Source: three-view drawing plus pictorial views. Frame: mm from the lowest corner of the part. A direction names the side the tool comes from. Give positions to 0.01 mm unless a question says otherwise; leave off trailing zeros. Order: outer loops, then holes, each group sorted by start corner. A loop starts at its lowest first (then second) coordinate and runs counter-clockwise, first axis right, second up. Notation, with made-up numbers: M 25,-22.5 L 67,-22.5 A5 ccw 67,-16.5 Z; hole C 59.25,24 d2. An arc over 180 degrees is marked long. Use CSV: the item, a comma, the result in double quotes.
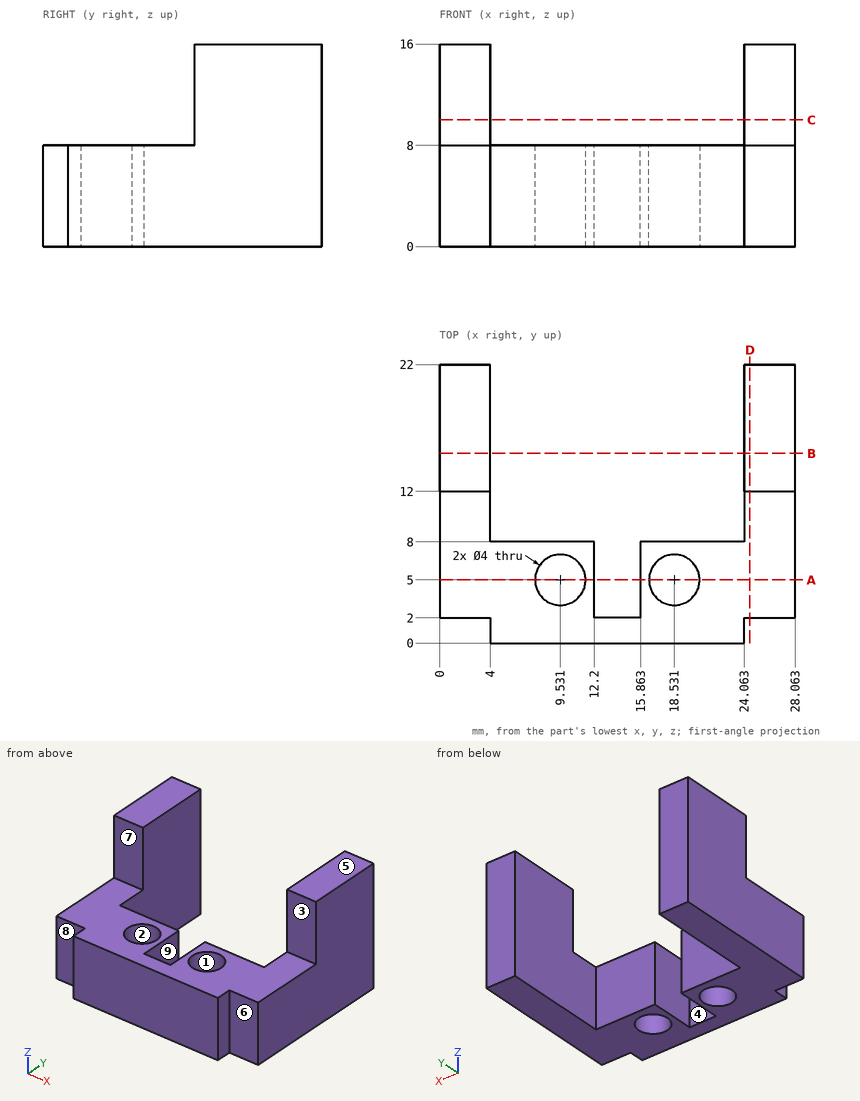
1. Section C-C, the plane z = 10. Return the cut outline in (x, y).
Answer:
outline,"M 0,12 L 4,12 L 4,22 L 0,22 Z; M 24.06,12 L 28.06,12 L 28.06,22 L 24.06,22 Z"
2. Section A-A, the plane y = 5. Return the cut outline in (x, z), plus the area to 3 significant figures.
Answer:
outline,"M 0,0 L 7.53,0 L 7.53,8 L 0,8 Z; M 11.53,0 L 12.2,0 L 12.2,8 L 11.53,8 Z; M 15.86,0 L 16.53,0 L 16.53,8 L 15.86,8 Z; M 20.53,0 L 28.06,0 L 28.06,8 L 20.53,8 Z"
area,"131 mm2"
3. Reachability of the marked faces 5, 6, 7, 8 and 9 from +Z, -Z, +X, -X, +Y, -Y: full face, straight path, thin tool, end or side. Return the list, or none.
Answer:
face 5,"+Z, +X, -X, +Y, -Y"
face 6,"+Z, -Z, +X, -Y"
face 7,"+Z, +X, -X, -Y"
face 8,"+Z, -Z, -X, -Y"
face 9,"+Z, -Z, +Y"
4. Pin query (flat end, axial travel): pin 1 Ø3 at (x, z) = (26, 5) entering from -Y; pin 2 Ø6.5 at (x, y) = (18.53, 5) entering from +Z; pin 3 Ø1.8 at (y, z) = (6, 4.5) entering from -X; pin 4 Ø1.8 at (x, z) = (14, 2) entering from +Y. Return the tip coordinate at first contact, or that it passes through.
Answer:
pin 1,"y = 2"
pin 2,"z = 8"
pin 3,"x = 0"
pin 4,"y = 2"
5. Line query: line 1 (X direction, y = 16.5, z = 11.5); line 2 (X direction, y = 4.25, z = 5.25) (1 decimal); line 3 (Y direction, x = 14, z = 1). Output: solid intervals per line, ascending.
Answer:
line 1,"0 to 4, 24.06 to 28.06"
line 2,"0 to 7.7, 11.4 to 12.2, 15.9 to 16.7, 20.4 to 28.1"
line 3,"0 to 2"
6. Pull-direction query (Y, two-part tool) for the marked faces 1, 2, 3 and 4; classes: +Y half, -Y half, draft (parallel to the pull), parting line (faces both ways), or undercut.
Answer:
face 1,"undercut"
face 2,"undercut"
face 3,"-Y half"
face 4,"+Y half"
7. Section B-B, the plane y = 15. Return the cut outline in (x, z), plus the area to 3 significant figures.
Answer:
outline,"M 0,0 L 4,0 L 4,16 L 0,16 Z; M 24.06,0 L 28.06,0 L 28.06,16 L 24.06,16 Z"
area,"128 mm2"
8. Section D-D, the plane x = 24.5. Return the cut outline in (y, z), plus the area to 3 significant figures.
Answer:
outline,"M 2,0 L 22,0 L 22,16 L 12,16 L 12,8 L 2,8 Z"
area,"240 mm2"
